from build123d import *

# Parameters (mm, degrees)
SKETCH1_W                  = 107.7
SKETCH1_H                  = 50
BOSS_EXTRUDE1_DEPTH        = 40
SKETCH2_W                  = 75.7
SKETCH2_H                  = 40
CUT_EXTRUDE1_DEPTH         = 35
CUT_EXTRUDE2_REACH         = 125.791
SKETCH4_W                  = 19.6
SKETCH4_H                  = 40
SKETCH5_W                  = 45
SKETCH5_H                  = 10.3
CUT_EXTRUDE3_DEPTH         = 126.296807621
M4X0_7_TAPPED_HOLE1_D      = 3.3
F_3_0MM_DOWEL_HOLE1_D      = 3
F_3_0MM_DOWEL_HOLE1_DEPTH  = 7
F_3_0MM_DOWEL_HOLE2_D      = 3
F_3_0MM_DOWEL_HOLE2_DEPTH  = 7
M3X0_5_TAPPED_HOLE1_D      = 2.5
M3X0_5_TAPPED_HOLE1_DEPTH  = 7.5
M3X0_5_TAPPED_HOLE1_TIP    = 0.751075774
F_3_0MM_DOWEL_HOLE3_D      = 3
HOLE1_D                    = 16
HOLE1_DEPTH                = 7
M3X0_5_TAPPED_HOLE2_D      = 2.5
M3X0_5_TAPPED_HOLE2_DEPTH  = 7.5
M3X0_5_TAPPED_HOLE2_TIP    = 0.751075774
F_3_0MM_DOWEL_HOLE4_D      = 3
M3X0_5_TAPPED_HOLE3_D      = 2.5
M3X0_5_TAPPED_HOLE3_DEPTH  = 7.5
M3X0_5_TAPPED_HOLE3_TIP    = 0.751075774
M3X0_5_TAPPED_HOLE4_REACH  = 127.297
M3X0_5_TAPPED_HOLE4_BORE_R = 1.25
F_1_1_DIAMETER_HOLE1_D     = 25.4
F_1_1_DIAMETER_HOLE1_DEPTH = 25
M4X0_7_TAPPED_HOLE2_D      = 3.3
M4X0_7_TAPPED_HOLE2_DEPTH  = 7.407641206
M3X0_5_TAPPED_HOLE5_D      = 2.5
M3X0_5_TAPPED_HOLE5_DEPTH  = 5
M3X0_5_TAPPED_HOLE5_TIP    = 0.751075774
FILLET1_R                  = 2
FILLET2_R                  = 3
FILLET3_R                  = 10
SKETCH32_R                 = 2.5
CUT_EXTRUDE4_DEPTH         = 5
M2X0_4_TAPPED_HOLE1_D      = 1.6
M2X0_4_TAPPED_HOLE1_DEPTH  = 5.2
M2X0_4_TAPPED_HOLE1_TIP    = 0.480688495


with BuildPart() as part:
    # Sketch1 → Boss-Extrude1 (new body)
    with BuildSketch(Plane.XY.offset(40)):
        with Locations((53.85, -25)):
            Rectangle(SKETCH1_W, SKETCH1_H)
    extrude(amount=-BOSS_EXTRUDE1_DEPTH)

    # Sketch2 → Cut-Extrude1 (cut)
    with BuildSketch(Plane.XY.offset(40)):
        with Locations((62.85, -25)):
            Rectangle(SKETCH2_W, SKETCH2_H)
    extrude(amount=-CUT_EXTRUDE1_DEPTH, mode=Mode.SUBTRACT)

    # Sketch4 → Cut-Extrude2 (cut, up to next)
    with BuildSketch(Plane(origin=(0, 0, 35), x_dir=(-1, 0, 0), z_dir=(0, 0, -1)), mode=Mode.PRIVATE) as cut_extrude2_sk1:
        with Locations((-15.2, -25)):
            Rectangle(SKETCH4_W, SKETCH4_H)
    cut_extrude2_tool1 = extrude(cut_extrude2_sk1.sketch, amount=-CUT_EXTRUDE2_REACH, mode=Mode.PRIVATE) & part.part
    add(cut_extrude2_tool1.solids().sort_by_distance((15.2, -25, 35))[0], mode=Mode.SUBTRACT)

    # Sketch5 → Cut-Extrude3 (cut, through all)
    with BuildSketch(Plane(origin=(0, 0, 0), x_dir=(-1, 0, 0), z_dir=(0, 0, -1))):
        with Locations((-77.2, -25)):
            Rectangle(SKETCH5_W, SKETCH5_H)
    extrude(amount=-CUT_EXTRUDE3_DEPTH, mode=Mode.SUBTRACT)

    # M4x0.7 Tapped Hole1 (through all)
    with Locations(Plane(origin=(0, 0, 0), x_dir=(-1, 0, 0), z_dir=(0, 0, -1))):
        with Locations((-58, -42), (-78, -42), (-98, -42), (-98, -8), (-58, -8), (-78, -8)):
            Hole(M4X0_7_TAPPED_HOLE1_D / 2)

    # Ø3.0mm Dowel Hole1
    with Locations(Plane.ZY.offset(-100.7)):
        with Locations((11, -11)):
            Hole(F_3_0MM_DOWEL_HOLE1_D / 2, depth=F_3_0MM_DOWEL_HOLE1_DEPTH)

    # Ø3.0mm Dowel Hole2
    with Locations(Plane(origin=(107.7, 0, 0), x_dir=(0, 0, -1), z_dir=(1, 0, 0))):
        with Locations((-29, -39)):
            Hole(F_3_0MM_DOWEL_HOLE2_D / 2, depth=F_3_0MM_DOWEL_HOLE2_DEPTH)

    # M3x0.5 Tapped Hole1
    with Locations(Plane(origin=(0, 0, 0), x_dir=(1, 0, 0), z_dir=(0, 1, 0))):
        with Locations((22.5, -11)):
            Hole(M3X0_5_TAPPED_HOLE1_D / 2, depth=M3X0_5_TAPPED_HOLE1_DEPTH)
            with Locations((0, 0, -(M3X0_5_TAPPED_HOLE1_DEPTH + M3X0_5_TAPPED_HOLE1_TIP / 2))):  # 118° drill point
                Cone(0, M3X0_5_TAPPED_HOLE1_D / 2, M3X0_5_TAPPED_HOLE1_TIP, mode=Mode.SUBTRACT)

    # Ø3.0mm Dowel Hole3 (through all)
    with Locations(Plane(origin=(25, 0, 0), x_dir=(0, 0, -1), z_dir=(1, 0, 0))):
        with Locations((-11, -11)):
            Hole(F_3_0MM_DOWEL_HOLE3_D / 2)

    # Hole1
    with Locations(Plane.ZY.offset(-100.7)):
        with Locations((20, -25)):
            Hole(HOLE1_D / 2, depth=HOLE1_DEPTH)

    # M3x0.5 Tapped Hole2
    with Locations(Plane.XY.offset(40)):
        with Locations((104.2, -25)):
            Hole(M3X0_5_TAPPED_HOLE2_D / 2, depth=M3X0_5_TAPPED_HOLE2_DEPTH)
            with Locations((0, 0, -(M3X0_5_TAPPED_HOLE2_DEPTH + M3X0_5_TAPPED_HOLE2_TIP / 2))):  # 118° drill point
                Cone(0, M3X0_5_TAPPED_HOLE2_D / 2, M3X0_5_TAPPED_HOLE2_TIP, mode=Mode.SUBTRACT)

    # Ø3.0mm Dowel Hole4 (through all)
    with Locations(Plane.ZY):
        with Locations((29, -39)):
            Hole(F_3_0MM_DOWEL_HOLE4_D / 2)

    # M3x0.5 Tapped Hole3
    with Locations(Plane.XY.offset(40)):
        with Locations((2.9, -37), (93.85, -2.5), (53.85, -2.5), (13.85, -2.5), (2.9, -13), (13.85, -47.5), (53.85, -47.5), (93.85, -47.5)):
            Hole(M3X0_5_TAPPED_HOLE3_D / 2, depth=M3X0_5_TAPPED_HOLE3_DEPTH)
            with Locations((0, 0, -(M3X0_5_TAPPED_HOLE3_DEPTH + M3X0_5_TAPPED_HOLE3_TIP / 2))):  # 118° drill point
                Cone(0, M3X0_5_TAPPED_HOLE3_D / 2, M3X0_5_TAPPED_HOLE3_TIP, mode=Mode.SUBTRACT)

    # M3x0.5 Tapped Hole4 bore → M3x0.5 Tapped Hole4 (cut, up to next)
    with BuildSketch(Plane(origin=(0, -50, 0), x_dir=(-1, 0, 0), z_dir=(0, -1, 0)), mode=Mode.PRIVATE) as m3x0_5_tapped_hole4_sk1:
        with Locations((-22.5, -29)):
            Circle(M3X0_5_TAPPED_HOLE4_BORE_R)
    m3x0_5_tapped_hole4_tool1 = extrude(m3x0_5_tapped_hole4_sk1.sketch, amount=-M3X0_5_TAPPED_HOLE4_REACH, mode=Mode.PRIVATE) & part.part
    add(m3x0_5_tapped_hole4_tool1.solids().sort_by_distance((22.5, -50, 29))[0], mode=Mode.SUBTRACT)

    # 1 (1) Diameter Hole1
    with Locations(Plane.ZY):
        with Locations((20, -25)):
            Hole(F_1_1_DIAMETER_HOLE1_D / 2, depth=F_1_1_DIAMETER_HOLE1_DEPTH)

    # M4x0.7 Tapped Hole2
    with Locations(Plane(origin=(0, 0, 32.592358794), x_dir=(-1, 0, 0), z_dir=(0, 0, -1))):
        with Locations((-7, -25)):
            Hole(M4X0_7_TAPPED_HOLE2_D / 2, depth=M4X0_7_TAPPED_HOLE2_DEPTH)

    # M3x0.5 Tapped Hole5
    with Locations(Plane.XY.offset(35)):
        with Locations((19.5, -10), (19.5, -40)):
            Hole(M3X0_5_TAPPED_HOLE5_D / 2, depth=M3X0_5_TAPPED_HOLE5_DEPTH)
            with Locations((0, 0, -(M3X0_5_TAPPED_HOLE5_DEPTH + M3X0_5_TAPPED_HOLE5_TIP / 2))):  # 118° drill point
                Cone(0, M3X0_5_TAPPED_HOLE5_D / 2, M3X0_5_TAPPED_HOLE5_TIP, mode=Mode.SUBTRACT)

    # Fillet1
    fillet1_edges = [part.edges().sort_by_distance(p)[0] for p in [
        (100.7, -45, 22.5),
        (25, -45, 20),
        (25, -5, 20),
        (100.7, -5, 22.5),
        (99.7, -30.15, 2.5),
        (99.7, -19.85, 2.5),
        (54.7, -19.85, 2.5),
        (54.7, -30.15, 2.5),
    ]]
    fillet(fillet1_edges, radius=FILLET1_R)

    # Fillet2
    fillet2_edges = [part.edges().sort_by_distance(p)[0] for p in [
        (5.4, -45, 37.5),
        (5.4, -5, 37.5),
    ]]
    fillet(fillet2_edges, radius=FILLET2_R)

    # Fillet3
    # the kernel refuses this fillet: 10 mm, written as the material it takes off along each edge
    with BuildSketch(Plane(origin=(0, 0, 65), x_dir=(0, -1, 0), z_dir=(0, 0, -1)), Plane(origin=(0, -50, 65), x_dir=(1, 0, 0), z_dir=(0, 0, -1))) as fillet3_piece_1:
        with BuildLine():
            CenterArc((FILLET3_R, -FILLET3_R), FILLET3_R, 90, 90)
            Line((0, -FILLET3_R), (0, 0))
            Line((0, 0), (FILLET3_R, 0))
        make_face()
    extrude(amount=90, mode=Mode.SUBTRACT)
    with BuildSketch(Plane(origin=(107.7, 0, 65), x_dir=(0, -1, 0), z_dir=(0, 0, -1)), Plane(origin=(107.7, -50, 65), x_dir=(-1, 0, 0), z_dir=(0, 0, -1))) as fillet3_piece_2:
        with BuildLine():
            CenterArc((FILLET3_R, FILLET3_R), FILLET3_R, 180, 90)
            Line((0, FILLET3_R), (0, 0))
            Line((0, 0), (FILLET3_R, 0))
        make_face()
    extrude(amount=90, mode=Mode.SUBTRACT)

    # Sketch32 → Cut-Extrude4 (cut)
    with BuildSketch(Plane.XY.offset(40)):
        with Locations((7, -25)):
            Circle(SKETCH32_R)
    extrude(amount=-CUT_EXTRUDE4_DEPTH, mode=Mode.SUBTRACT)

    # M2x0.4 Tapped Hole1
    with Locations(Plane(origin=(0, -45, 0), x_dir=(1, 0, 0), z_dir=(0, 1, 0))):
        with Locations((33.7, -36.5), (48.7, -36.5), (63.7, -36.5), (78.7, -36.5)):
            Hole(M2X0_4_TAPPED_HOLE1_D / 2, depth=M2X0_4_TAPPED_HOLE1_DEPTH)
            with Locations((0, 0, -(M2X0_4_TAPPED_HOLE1_DEPTH + M2X0_4_TAPPED_HOLE1_TIP / 2))):  # 118° drill point
                Cone(0, M2X0_4_TAPPED_HOLE1_D / 2, M2X0_4_TAPPED_HOLE1_TIP, mode=Mode.SUBTRACT)


solid = part.part
Work out the finished part from the listing and answer in its coordinate system (mm). A direction names the side the tool comes from. Give positions to 0.01 mm unless a question says otherwise; leave off trailing zeros. Write each loop counter-clockwise with the first axis right and the second up, starting at its lowest first coordinate (ties: lowest second). Pieces come first, ordered by that corner, then holes. Notation, with made-up numbers: M -15.5,38.25 L 37.5,38.25 A29 cw 37.5,61.25 Z; hole C -26.5,32 d7. An arc over 180 degrees is marked long. Answer as CSV lines item,"result".
Q1. A cutting plane is placed at B-B on x = 75. Write down the section's boundary in (y, z).
A:
outline,"M -50,0 L -30.15,0 L -30.15,5 L -45,5 L -45,40 L -50,40 Z; M -19.85,0 L 0,0 L 0,40 L -5,40 L -5,5 L -19.85,5 Z"
Q2. A cutting plane is placed at A-A on z = 20. Write down the section's boundary in (x, y).
A:
outline,"M 0,-40 A10 ccw 10,-50 L 97.7,-50 A10 ccw 107.7,-40 L 107.7,-33 L 100.7,-33 L 100.7,-43 A2 cw 98.7,-45 L 27,-45 A2 cw 25,-43 L 25,-37.7 L 0,-37.7 Z; M 0,-12.3 L 25,-12.3 L 25,-7 A2 cw 27,-5 L 98.7,-5 A2 cw 100.7,-7 L 100.7,-17 L 107.7,-17 L 107.7,-10 A10 ccw 97.7,0 L 10,0 A10 ccw 0,-10 Z"
Q3. Given P1, Ø1, axis at x = 65, z = 26.5, coming from the +Y side; P2, Ø3, axis at x = 19.5, y = -40, coming from the +Z side; P3, Ø1.5, axis at x = 53.85, y = -47.5, coming from the +Z side; P4, Ø2, axis at x = 19.5, y = -10, coming from the +Z side, each flat-ended and moving along its own axis, determine where each tip first touches the part or whether it passes through.
A:
P1,"stops at y = 0"
P2,"stops at z = 35"
P3,"stops at z = 32.2"
P4,"stops at z = 29.85"
Q4. A cutting plane is placed at C-C on y = -34.5. Write down the section's boundary in (x, z).
A:
outline,"M 0,0 L 107.7,0 L 107.7,40 L 100.7,40 L 100.7,5 L 25,5 L 25,11.57 L 0,11.57 Z; M 0,28.43 L 25,28.43 L 25,35 L 5.4,35 L 5.4,40 L 0,40 Z"
Q5. A cutting plane is placed at D-D on z = 3.5. Write down the section's boundary in (x, y).
A:
outline,"M 0,-40 A10 ccw 10,-50 L 97.7,-50 A10 ccw 107.7,-40 L 107.7,-10 A10 ccw 97.7,0 L 10,0 A10 ccw 0,-10 Z; hole M 54.7,-28.15 A2 ccw 56.7,-30.15 L 97.7,-30.15 A2 ccw 99.7,-28.15 L 99.7,-21.85 A2 ccw 97.7,-19.85 L 56.7,-19.85 A2 ccw 54.7,-21.85 Z; hole C 58,-42 d3.3; hole C 58,-8 d3.3; hole C 78,-42 d3.3; hole C 78,-8 d3.3; hole C 98,-42 d3.3; hole C 98,-8 d3.3"
Q6. The mould has two halves that part along X. Classify faces 5 (the cylindrical face through (104.2, -11.9, 12.2)), 6 (the conical face through (2.872, -12.785, 31.879)), 7 (the cylindrical face through (100.13, -44.4, 22.26)): +X half, -X half, draft (parallel to the pull), parting line (faces both ways), or undercut.
A:
face 5,"draft"
face 6,"undercut"
face 7,"undercut"
Q7. Find the intervals of material crossed by probe 1 along Y at (x, z) = (58, 2); probe 2 along Y at (x, z) = (14, 33); probe 3 along Y at (x, z) = (53, 19), in increasing order. Write a range as [from, to].
A:
probe 1,"y = [-50, -43.65], [-40.35, -30.15], [-19.85, -9.65], [-6.35, 0]"
probe 2,"y = [-50, -48.74], [-46.26, -3.74], [-1.26, 0]"
probe 3,"y = [-50, -45], [-5, 0]"
Q8. A tool of negligible diameter and unlimited length cuts with its end or side. For faces 1 (the cylindrical face through (21.31, -44.99, 28.62)), 2 (the flat face through (99.7, -25, 2)), 3 (the flat face through (16, -25, 35)), 4 (the flat face through (53, -25, 0)), from which of +Z, -Z, +X, -X, +Y, -Y can it reach the whole face along a straight path? Write none if from no direction.
A:
face 1,"-Y"
face 2,"+Z, -Z"
face 3,"+Z"
face 4,"-Z, +X, -X, +Y, -Y"
